```python
from build123d import *

# Parameters (mm, degrees)
F1_DEPTH = 7.62
F2_R     = 12.7
F2_R_2   = 9.398
F3_DEPTH = 31.75
F4_R     = 12.7
F4_R_2   = 11.176
F5_DEPTH = 12.7
F6_R     = 6.35
F7_DEPTH = 25.4
F8_R     = 0.762
F9_SIZE2 = 0.508
F9_SIZE  = 0.8798818102


with BuildPart() as f1:
    # F0 (on Front) → F1 (new body)
    with BuildSketch(Plane.XZ):
        with BuildLine():
            ThreePointArc((-21.1420084076, -2.54), (-20.3980596318, -0.7439487758), (-18.6020084076, 0))
            Line((-18.6020084076, 0), (32.7059915924, 0))
            ThreePointArc((32.7059915924, 0), (35.4000684287, -1.1159231637), (36.5159915924, -3.81))
            Line((36.5159915924, -3.81), (36.5159915924, -8.89))
            Line((36.5159915924, -8.89), (34.3569915924, -8.89))
            Line((34.3569915924, -8.89), (34.3569915924, -4.318))
            ThreePointArc((34.3569915924, -4.318), (33.6874376942, -2.7015538982), (32.0709915924, -2.032))
            Line((32.0709915924, -2.032), (29.2769915924, -2.032))
            Line((29.2769915924, -2.032), (17.8469915924, -2.032))
            Line((17.8469915924, -2.032), (17.8469915924, -9.652))
            Line((17.8469915924, -9.652), (24.7049915924, -9.652))
            ThreePointArc((24.7049915924, -9.652), (27.937883796, -10.9911077964), (29.2769915924, -14.224))
            Line((29.2769915924, -14.224), (29.2769915924, -15.24))
            ThreePointArc((29.2769915924, -15.24), (29.6489659803, -16.1380256121), (30.5469915924, -16.51))
            Line((30.5469915924, -16.51), (42.8659915924, -16.51))
            ThreePointArc((42.8659915924, -16.51), (43.7640172045, -16.1380256121), (44.1359915924, -15.24))
            Line((44.1359915924, -15.24), (44.1359915924, 0))
            Line((44.1359915924, 0), (12.7, 127))
            ThreePointArc((12.7, 127), (0, 139.7), (-12.7, 127))
            Line((-12.7, 127), (-31.3020084076, 0))
            Line((-31.3020084076, 0), (-31.3020084076, -16.51))
            ThreePointArc((-31.3020084076, -16.51), (-30.9300340197, -17.4080256121), (-30.0320084076, -17.78))
            Line((-30.0320084076, -17.78), (-22.4120084076, -17.78))
            ThreePointArc((-22.4120084076, -17.78), (-21.5139827955, -17.4080256121), (-21.1420084076, -16.51))
            Line((-21.1420084076, -16.51), (-21.1420084076, -2.54))
        make_face()
        Polygon((13.8583155349, 10.2559253573), (-17.4904800951, 10.2559253573), (-17.9861974368, 10.2559253573), (-16.4103638381, 24.8740110546), align=None, mode=Mode.SUBTRACT)
        Polygon((30.8991490559, 10.2559253573), (-15.5502194539, 32.8530669212), (18.8005114427, 63.1991239488), align=None, mode=Mode.SUBTRACT)
        Polygon((16.8689347681, 72.4665825348), (-14.2382610105, 45.0233372929), (-10.1512422372, 82.9362176403), align=None, mode=Mode.SUBTRACT)
        Polygon((-7.1419274588, 110.8518689871), (8.8684540242, 110.8518689871), (14.6986516415, 82.8793242388), (-9.1010310551, 92.6784119132), align=None, mode=Mode.SUBTRACT)
    extrude(amount=F1_DEPTH)

    # F2 (on face) → F3 (join)
    with BuildSketch(Plane.XZ.offset(7.62)):
        with Locations((0, 127)):
            Circle(F2_R)
        with Locations((0, 127)):
            Circle(F2_R_2, mode=Mode.SUBTRACT)
    extrude(amount=F3_DEPTH)

    # F4 (on face) → F5 (join)
    with BuildSketch(Plane.XZ.offset(39.37)):
        with Locations((0, 127)):
            Circle(F4_R)
        with Locations((0, 127)):
            Circle(F4_R_2, mode=Mode.SUBTRACT)
    extrude(amount=F5_DEPTH)

    # F6 (on face) → F7 (cut)
    with BuildSketch(Plane.XZ.offset(7.62)):
        with Locations((0, 127)):
            Circle(F6_R)
    extrude(amount=-F7_DEPTH, mode=Mode.SUBTRACT)

    # F8
    f8_edges = [f1.edges().sort_by_distance(p)[0] for p in [
        (-11.176, -52.07, 127),
    ]]
    fillet(f8_edges, radius=F8_R)

    # F9
    f9_edges = [f1.edges().sort_by_distance(p)[0] for p in [
        (-31.302008, 0, -8.255),
        (-22.001004, 0, 63.5),
        (-30.930034, 0, -17.408026),
        (0, 0, 139.7),
        (-26.222008, 0, -17.78),
        (28.417996, 0, 63.5),
        (-21.513983, 0, -17.408026),
        (44.135992, 0, -7.62),
        (-21.142008, 0, -9.525),
        (43.764017, 0, -16.138026),
        (-20.39806, 0, -0.743949),
        (36.706492, 0, -16.51),
        (7.051992, 0, 0),
        (29.648966, 0, -16.138026),
        (35.400068, 0, -1.115923),
        (29.276992, 0, -14.732),
        (36.515992, 0, -6.35),
        (27.937884, 0, -10.991108),
        (35.436492, 0, -8.89),
        (21.275992, 0, -9.652),
        (34.356992, 0, -6.604),
        (17.846992, 0, -5.842),
        (33.687438, 0, -2.701554),
        (24.958992, 0, -2.032),
        (-17.198281, 0, 17.564968),
        (-2.063941, 0, 10.255925),
        (-1.276024, 0, 17.564968),
        (1.315337, 0, 58.74496),
        (3.358846, 0, 77.7014),
        (-12.194752, 0, 63.979777),
        (24.84983, 0, 36.727525),
        (1.625146, 0, 48.026095),
        (7.674465, 0, 21.554496),
        (0.863263, 0, 110.851869),
        (-8.121479, 0, 101.76514),
        (11.783553, 0, 96.865597),
        (2.79881, 0, 87.778868),
        (-6.35, 0, 127),
    ]]
    f9_side = f1.faces().sort_by_distance((-29.555846, 0, -8.255))[0]
    chamfer(f9_edges, length=F9_SIZE, length2=F9_SIZE2, reference=f9_side)


solid = f1.part
```
Input: part model. Units: mm. Frame: model coordinates. A direction names the side the tool comes from. Coordinates: 2 decimals unless noted, no trailing zeros. Loops run counter-clockwise (first coordinate to the right, second up) from the corner with the lowest first, then second, coordinate; pieces in that order, holes last. Notation, with made-up numbers: M 17.5,-19.5 L 25.5,-19.5 A30 ccw 25.5,17.5 Z; hole C 67,35.25 d10. An arc over 180 degrees is marked long. One line per item, written item: value.
(1) Section A-A (z = 13). Output: boundary loops of the cut face in (x, y).
Filled in:
outline: M -29.4,-7.62 L -17.69,-7.62 L -17.69,-0.51 L -18.58,0 L -28.51,0 L -29.4,-0.51 Z; M 8.18,-7.62 L 25.26,-7.62 L 25.26,-0.51 L 23.25,0 L 10.2,0 L 8.18,-0.51 Z; M 30.27,-7.62 L 40.92,-7.62 L 40.92,-0.51 L 40.01,0 L 31.17,0 L 30.27,-0.51 Z
(2) Reachability of faces 1 (the flat face through (-21.44, -0.26, 64.36)), 2 (the flat face through (-21.87, -4.01, 64.39)), 3 (the flat face through (37, -4, -16.51)), 4 (the flat face through (-17.21, -4.01, 17.46)), 5 (the flat face through (-0.162, -0.258, 17.509)) from +Z, -Z, +X, -X, +Y, -Y: full face, straight path, thin tool, end or side. Return the list, or none.
Filled in:
face 1: +Z, -X, +Y
face 2: +Z, -X, +Y, -Y
face 3: -Z, +X, +Y, -Y
face 4: +Y, -Y
face 5: +Y
(3) Section D-D (x = 0). Give the number of separate pieces and of enclosed holes in the cut face, and give its area (3 significant figures).
Filled in:
separate pieces: 6
enclosed holes: 0
area: 669 mm^2
(4) Line query: line 1 along Z through (x, y) = (0, -27); line 2 along Z through (x, y) = (0, -45.5); line 3 along Z through (x, y) = (0, -4). Output: solid intervals per line, ascending. Write a range as from..to.
Filled in:
line 1: 114.3..117.6, 136.4..139.7
line 2: 114.3..115.82, 138.18..139.7
line 3: 0..10.26, 16.95..25.29, 46.59..57.58, 79..88.93, 110.85..120.65, 133.35..139.7
(5) Pin query (flat end, axial travel): pin 1 (12 mm diameter, centred on x = 21.5, z = 84, fed in from -Y); pin 2 (16.5 mm diameter, centred on x = 0, z = 127, fed in from +Y); pin 3 (10 mm diameter, centred on y = -9.5, z = 14, fed in from +X); pin 4 (5 mm diameter, centred on x = 1.5, y = -25.5, fed in from -Z). Return the tip coordinate at first contact, or that it passes through.
Filled in:
pin 1: y = -7.62
pin 2: y = 0
pin 3: x = 41.82
pin 4: z = 114.3
(6) Section B-B (z = 67.5). Output: boundary loops of the cut face in (x, y).
Filled in:
outline: M -21.42,-7.62 L -11.82,-7.62 L -11.82,-0.51 L -12.7,0 L -20.53,0 L -21.42,-0.51 Z; M 11.24,-7.62 L 27.43,-7.62 L 27.43,-0.51 L 26.52,0 L 12.57,0 L 11.24,-0.51 Z
(7) Pull-direction query (Z, two-part tool) for faces 6 (the flat face through (-26, -4, -17.78)), 7 (the flat face through (28.64, -4.01, 62.61)), 8 (the flat face through (1, -4, 110.852)), 9 (the flat face through (1.53, -0.26, 58.36)); classes: +Z half, -Z half, draft (parallel to the pull), parting line (faces both ways), or undercut.
Filled in:
face 6: -Z half
face 7: +Z half
face 8: undercut
face 9: undercut
(8) Section C-C (y = -25.5). Output: boundary loops of the cut face in (x, z), and give its area (3 significant figures).
Filled in:
outline: C 0,127 d25.4; hole C 0,127 d18.8
area: 229 mm^2
